Geometry: final body of the model. Coordinates: model frame, mm. Give positions to 0.01 mm unless a question says otherwise; leave off trailing zeros. Loops run counter-clockwise (first coordinate to the right, second up) from the corner with the lowest first, then second, coordinate; pieces in that order, holes last.
1. Section D-D, the plane z = 4. State how many separate pieces and enclosed holes the cut face has, then the cut area to 3 significant figures.
2. Section A-A, the plane x = 9.7. Output: boundary loops of the cut face in (y, z), then the cut area to 3 significant figures.
3. Section B-B, the plane y = 12.3. Output: boundary loops of the cut face in (x, z).
4. Material intervals for line 1 along Y through (x, z) = (6, 4.75); line 2 along X through (y, z) = (59, 3.5); line 3 along X through (y, z) = (-60.5, 1.25), sorted ascending.
5. Section C-C, the plane y = -60. Output: boundary loops of the cut face in (x, z).
6. Draft query along X for faces 1 (the face through (-30, 1, 3)), 2 (the face through (23.746, 61.933, 3.131)), 3 (the face through (0, 1, 6.35)). Return one class per face: +X half, -X half, draft (parallel to the pull), parting line (faces both ways), or undercut.
from build123d import *

# Parameters (mm, degrees)
SKETCH1_R           = 1.95
SKETCH1_R_2         = 2
BOSS_EXTRUDE1_DEPTH = 6.35


with BuildPart() as part:
    # Sketch1 → Boss-Extrude1 (new body)
    with BuildSketch(Plane.XY):
        with BuildLine():
            Line((-25, -67.5), (25, -67.5))
            ThreePointArc((25, -67.5), (28.535533906, -66.035533906), (30, -62.5))
            Line((30, -62.5), (30, 62.5))
            ThreePointArc((30, 62.5), (28.535533906, 66.035533906), (25, 67.5))
            Line((25, 67.5), (-25, 67.5))
            ThreePointArc((-25, 67.5), (-28.535533906, 66.035533906), (-30, 62.5))
            Line((-30, 62.5), (-30, -62.5))
            ThreePointArc((-30, -62.5), (-28.535533906, -66.035533906), (-25, -67.5))
        make_face()
        with Locations((24, 60)):
            Circle(SKETCH1_R, mode=Mode.SUBTRACT)
        with Locations((6, 60)):
            Circle(SKETCH1_R, mode=Mode.SUBTRACT)
        with Locations((6, 36.5)):
            Circle(SKETCH1_R, mode=Mode.SUBTRACT)
        with Locations((24, 36.5)):
            Circle(SKETCH1_R, mode=Mode.SUBTRACT)
        with Locations(Location((-6, 60, 0), (0, 0, 180))):
            Circle(SKETCH1_R, mode=Mode.SUBTRACT)
        with Locations(Location((-24, 60, 0), (0, 0, 180))):
            Circle(SKETCH1_R, mode=Mode.SUBTRACT)
        with Locations(Location((-24, 36.5, 0), (0, 0, 180))):
            Circle(SKETCH1_R, mode=Mode.SUBTRACT)
        with Locations(Location((-6, 36.5, 0), (0, 0, 180))):
            Circle(SKETCH1_R, mode=Mode.SUBTRACT)
        with Locations((-24, -36.5)):
            Circle(SKETCH1_R, mode=Mode.SUBTRACT)
        with Locations((-6, -36.5)):
            Circle(SKETCH1_R, mode=Mode.SUBTRACT)
        with Locations(Location((6, -36.5, 0), (0, 0, 180))):
            Circle(SKETCH1_R, mode=Mode.SUBTRACT)
        with Locations(Location((24, -36.5, 0), (0, 0, 180))):
            Circle(SKETCH1_R, mode=Mode.SUBTRACT)
        with Locations(Location((24, -60, 0), (0, 0, 180))):
            Circle(SKETCH1_R, mode=Mode.SUBTRACT)
        with Locations(Location((6, -60, 0), (0, 0, 180))):
            Circle(SKETCH1_R, mode=Mode.SUBTRACT)
        with Locations((-6, -60)):
            Circle(SKETCH1_R, mode=Mode.SUBTRACT)
        with Locations((-24, -60)):
            Circle(SKETCH1_R, mode=Mode.SUBTRACT)
        with Locations((9.7, -11.3)):
            Circle(SKETCH1_R_2, mode=Mode.SUBTRACT)
        with Locations((9.7, 12.3)):
            Circle(SKETCH1_R_2, mode=Mode.SUBTRACT)
        with Locations(Location((-9.7, -11.3, 0), (0, 0, 180))):
            Circle(SKETCH1_R_2, mode=Mode.SUBTRACT)
        with Locations(Location((-9.7, 12.3, 0), (0, 0, 180))):
            Circle(SKETCH1_R_2, mode=Mode.SUBTRACT)
    extrude(amount=BOSS_EXTRUDE1_DEPTH)


solid = part.part
Answers below:
1. separate pieces: 1
1. enclosed holes: 20
1. area: 7,840 mm2
2. outline: (-67.5, 0) - (-13.3, 0) - (-13.3, 6.35) - (-67.5, 6.35) - close; (-9.3, 0) - (10.3, 0) - (10.3, 6.35) - (-9.3, 6.35) - close; (14.3, 0) - (67.5, 0) - (67.5, 6.35) - (14.3, 6.35) - close
2. area: 806 mm2
3. outline: (-30, 0) - (-11.7, 0) - (-11.7, 6.35) - (-30, 6.35) - close; (-7.7, 0) - (7.7, 0) - (7.7, 6.35) - (-7.7, 6.35) - close; (11.7, 0) - (30, 0) - (30, 6.35) - (11.7, 6.35) - close
4. line 1: y = -67.5 to -61.95, -58.05 to -38.45, -34.55 to 34.55, 38.45 to 58.05, 61.95 to 67.5
4. line 2: x = -30 to -25.67, -22.33 to -7.67, -4.33 to 4.33, 7.67 to 22.33, 25.67 to 30
4. line 3: x = -30 to -25.88, -22.12 to -7.88, -4.12 to 4.12, 7.88 to 22.12, 25.88 to 30
5. outline: (-30, 0) - (-25.95, 0) - (-25.95, 6.35) - (-30, 6.35) - close; (-22.05, 0) - (-7.95, 0) - (-7.95, 6.35) - (-22.05, 6.35) - close; (-4.05, 0) - (4.05, 0) - (4.05, 6.35) - (-4.05, 6.35) - close; (7.95, 0) - (22.05, 0) - (22.05, 6.35) - (7.95, 6.35) - close; (25.95, 0) - (30, 0) - (30, 6.35) - (25.95, 6.35) - close
6. face 1: -X half
6. face 2: undercut
6. face 3: draft
